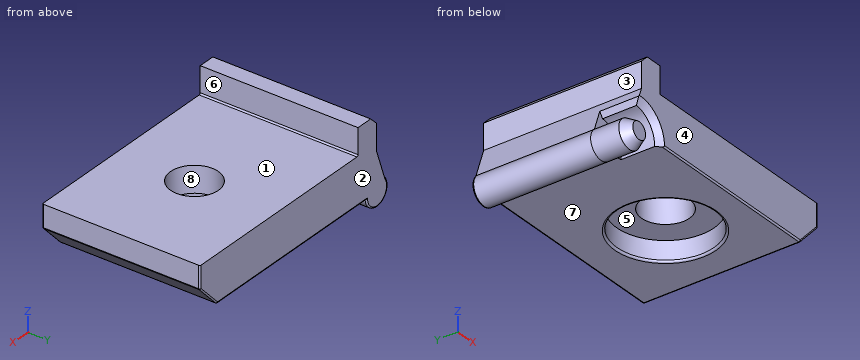
```python
from build123d import *

# Parameters (mm, degrees)
PAD007_DEPTH    = 28
SKETCH013_R     = 4.625
POCKET004_DEPTH = 7
SKETCH015_R     = 4.25
POCKET005_DEPTH = 49.001
SKETCH016_R     = 8.625
POCKET006_DEPTH = 4
CHAMFER_SIZE    = 1
FILLET007_R     = 0.25
FILLET008_R     = 0.35


with BuildPart() as part:
    # Sketch012 → Pad007 (new body)
    with BuildSketch(Plane(origin=(16, 14.5, -38.1), x_dir=(1, 0, 0), z_dir=(0, 1, 0))):
        with BuildLine():
            Line((0.5, 0.25), (37.5, 0.25))
            Line((37.5, 0.25), (37.5, 4.25))
            Line((33.5, 8.5), (37.5, 4.25))
            Line((33.5, 8.5), (-1.752001, 8.5))
            ThreePointArc((-1.752001, 8.5), (-5.341153, 10.649307), (-5.874808, 6.5))
            Line((-5.874808, 6.5), (-4.064, 1.4))
            Line((-4.064, 1.4), (-4.064, -3.148735))
            Line((-4.064, -3.148735), (-2.712735, -4.5))
            Line((-2.712735, -4.5), (0.25, -4.5))
            Line((0.25, -4.5), (0.25, 0))
            ThreePointArc((0.5, 0.25), (0.323223, 0.176777), (0.25, 0))
        make_face()
    extrude(amount=-PAD007_DEPTH)

    # Sketch013 → Pocket004 (cut)
    with BuildSketch(Plane.XZ.offset(6.5)):
        with Locations((11.75, -46.5)):
            Circle(SKETCH013_R)
    extrude(amount=POCKET004_DEPTH, mode=Mode.SUBTRACT)

    # Sketch014 → Revolution001 (revolve)
    with BuildSketch(Plane(origin=(11.75, -6.5, -46.5), x_dir=(0, 1, 0), z_dir=(1, 0, 0))):
        Polygon((-6.732051, 1.5), (-6.732051, 0), (0, 0), (0, 2.5), (-5, 2.5), align=None)
    revolve(axis=Axis((11.75, -6.5, -46.5), (0, 1, 0)))

    # Sketch015 → Pocket005 (cut, through all)
    with BuildSketch(Plane.XY):
        with Locations((35.55, 0)):
            Circle(SKETCH015_R)
    extrude(amount=-POCKET005_DEPTH, mode=Mode.SUBTRACT)

    # Sketch016 → Pocket006 (cut)
    with BuildSketch(Plane.XY.offset(-43)):
        with Locations((35.55, 0)):
            Circle(SKETCH016_R)
    extrude(amount=-POCKET006_DEPTH, mode=Mode.SUBTRACT)

    # Chamfer
    chamfer_edges = [part.edges().sort_by_distance(p)[0] for p in [
        (14.772373, -13.5, -42.999159),
        (11.075157, -10, -41.924499),
    ]]
    chamfer(chamfer_edges, length=CHAMFER_SIZE)

    # Fillet007
    fillet007_edges = [part.edges().sort_by_distance(p)[0] for p in [
        (33.437056, -13.5, -46.6),
        (51.5, -13.5, -44.475),
        (53.5, -13.5, -40.35),
        (53.5, 14.5, -40.35),
        (53.5, 0.5, -42.35),
        (51.5, 14.5, -44.475),
        (49.5, 0.5, -46.6),
        (31.874, 14.5, -46.6),
        (10.658847, 14.5, -48.749307),
    ]]
    fillet(fillet007_edges, radius=FILLET007_R)

    # Fillet008
    fillet008_edges = [part.edges().sort_by_distance(p)[0] for p in [
        (26.925, 0, -46.6),
    ]]
    fillet(fillet008_edges, radius=FILLET008_R)


solid = part.part
```
For this review, take the finished solid that the model builds, in its own axes (mm). Face numbers are marked on the shaded views. A direction names the side the tool comes from. Give positions to 0.01 mm unless a question says otherwise; leave off trailing zeros. Write each loop counter-clockwise with the first axis right and the second up, starting at its lowest first coordinate (ties: lowest second). Pieces come first, ordered by that corner, then holes. Notation, with made-up numbers: M 78,23 L 105,23 A22 cw 105,56 Z; hole C 61,14 d5. An arc over 180 degrees is marked long. Answer as a JSON object with one key per item and string values. Group by question number.
Item 1: Consider section D-D on z = -40. Write out the cut boundary in (x, y), plus the area to 3 significant figures.
Item 2: Draft analysis for pull direction X (two halves, no side actions). For the marked faces 6, 7 and 8, state which applies: +X half, -X half, draft (parallel to the pull), parting line (faces both ways), or undercut.
Item 3: Tool access review of the marked faces 1, 2, 3, 4 and 5: name each direction out of +Z, -Z, +X, -X, +Y, -Y from which nothing blocks a thin tool from reaching the whole face with its end or side.
Item 4: For pin 1 Ø1.5 at (x, z) = (12, -47) entering from -Y; pin 2 Ø1.7 at (x, z) = (14, -43) entering from -Y; pin 3 Ø3.5 at (y, z) = (-4, -36) entering from +X, all flat-tipped, find the tip position at first contact; note any pin that passes through.
Item 5: Consider section A-A on x = 35.55. Write out the cut boundary in (y, z) (3 decimals), plus the area to 3 significant figures.
Item 6: Consider section C-C on x = 23. Write out the cut boundary in (y, z), plus the area to 3 significant figures.
Item 7: Consider section B-B on y = 11.75. Write out the cut boundary in (x, z).
Item 8: For probe 1 along Y at (x, z) = (35.55, -42); probe 2 along Y at (x, z) = (35.55, -44.6) (3 decimals); probe 3 along Z at (x, y) = (47, -2.5), list the stretches that pass through material, from the lowest coordinate up. Write a range as [from, to].
Check result:
{
 "1": {"outline": "M 11.76,-13.5 L 53.25,-13.5 A0.25 ccw 53.5,-13.25 L 53.5,14.25 A0.25 ccw 53.25,14.5 L 11.76,14.5 Z; hole C 35.55,0 d8.5", "area": "1,110 mm^2"},
 "2": {"face 6": "+X half", "face 7": "draft", "face 8": "undercut"},
 "3": {"face 1": "+Z, +X, +Y, -Y", "face 2": "+Z, -Z, +X, -X, +Y", "face 3": "+Z, -X, +Y, -Y", "face 4": "+Z, -Z, +X, -X, -Y", "face 5": "-Z"},
 "4": {"pin 1": "stops at y = -13.23", "pin 2": "stops at y = -12.89", "pin 3": "stops at x = 16.25"},
 "5": {"outline": "M -13.5,-46.35 A0.25 ccw -13.25,-46.6 L -8.975,-46.6 A0.35 ccw -8.625,-46.25 L -8.625,-43 L -4.25,-43 L -4.25,-38.35 L -13.5,-38.35 Z; M 4.25,-43 L 8.625,-43 L 8.625,-46.25 A0.35 ccw 8.975,-46.6 L 14.25,-46.6 A0.25 ccw 14.5,-46.35 L 14.5,-38.35 L 4.25,-38.35 Z", "area": "129 mm^2"},
 "6": {"outline": "M -13.5,-46.35 A0.25 ccw -13.25,-46.6 L 14.25,-46.6 A0.25 ccw 14.5,-46.35 L 14.5,-38.35 L -13.5,-38.35 Z", "area": "231 mm^2"},
 "7": {"outline": "M 10.13,-44.6 A2.5 ccw long 14.25,-46.6 L 49.39,-46.6 A0.25 ccw 49.57,-46.52 L 53.43,-42.42 A0.25 ccw 53.5,-42.25 L 53.5,-38.35 L 16.5,-38.35 A0.25 cw 16.25,-38.1 L 16.25,-33.6 L 13.29,-33.6 L 11.94,-34.95 L 11.94,-39.5 Z"},
 "8": {"probe 1": "y = [-13.5, -4.25], [4.25, 14.5]", "probe 2": "y = [-13.5, -8.625], [8.625, 14.5]", "probe 3": "z = [-46.6, -38.35]"}
}
